```python
from build123d import *

# Parameters (mm, degrees)
BASPROSKE_W                  = 8
BASPROSKE_H                  = 13
TOOTHCUT_DEPTH               = 21.049937656
TEETHCUTS_COUNT              = 11
TEETHCUTS_ANGLE              = 327.272727273
BORSKE_R                     = 0.4
BORE_DEPTH                   = 50.0000508
ESTRUSIONE_ESTRUSIONE1_START = 10
SCHIZZO2_R                   = 13
ESTRUSIONE_ESTRUSIONE1_DEPTH = 10
TAGLIO_ESTRUSIONE1_DEPTH     = 14
FORO_PER_VITE_M3_1_D         = 4.2
FORO_PER_VITE_M3_1_DEPTH     = 9
FORO_PER_VITE_M3_1_TIP       = 1.2618073
SCHIZZO5_R                   = 11
TAGLIO_ESTRUSIONE2_DEPTH     = 2


with BuildPart() as part:
    # BasProSke → Base-Revolve (revolve)
    with BuildSketch(Plane(origin=(0, 0, 0), x_dir=(1, 0, 0), z_dir=(0, 1, 0)), mode=Mode.PRIVATE) as base_revolve_sk:
        with Locations((4, 6.5)):
            Rectangle(BASPROSKE_W, BASPROSKE_H)
    revolve(base_revolve_sk.sketch.rotate(Axis((-10, 0, 0), (1, 0, 0)), 180), axis=Axis((-10, 0, 0), (1, 0, 0)))

    # TooCutSke → ToothCut (cut, through all)
    with BuildSketch(Plane(origin=(0, 0, 0), x_dir=(0, 0, -1), z_dir=(1, 0, 0))):
        with BuildLine():
            ThreePointArc((1.139858048, 8.422216135), (0, 8.499), (-1.139858048, 8.422216135))
            ThreePointArc((-1.139858048, 8.422216135), (-1.658602184, 10.826907356), (-3.387115532, 12.577300725))
            ThreePointArc((-3.387115532, 12.577300725), (0, 13.0254), (3.387115532, 12.577300725))
            ThreePointArc((3.387115532, 12.577300725), (1.658602184, 10.826907356), (1.139858048, 8.422216135))
        make_face()
    toothcut = extrude(amount=TOOTHCUT_DEPTH, mode=Mode.SUBTRACT)

    # TeethCuts: ToothCut ×11 about axis
    teethcuts_axis = Axis((-10, 0, 0), (1, 0, 0))
    for i in range(1, TEETHCUTS_COUNT):
        add(toothcut.rotate(teethcuts_axis, i * TEETHCUTS_ANGLE / (TEETHCUTS_COUNT - 1)), mode=Mode.SUBTRACT)

    # BorSke → Bore (cut, symmetric)
    with BuildSketch(Plane(origin=(0, 0, 0), x_dir=(0, 0, -1), z_dir=(1, 0, 0))):
        with Locations(Location((0, 0, 0), (0, 0, 180))):
            Circle(BORSKE_R)
    extrude(amount=BORE_DEPTH, both=True, mode=Mode.SUBTRACT)

    # Schizzo2 → Estrusione-Estrusione1 (add)
    with BuildSketch(Plane(origin=(8, 0, 0), x_dir=(0, 0, -1), z_dir=(1, 0, 0)).offset(ESTRUSIONE_ESTRUSIONE1_START)):
        with Locations(Location((0, 0, 0), (0, 0, 173.223714884))):
            Circle(SCHIZZO2_R)
    extrude(amount=-ESTRUSIONE_ESTRUSIONE1_DEPTH)

    # Schizzo1 → Taglio-Estrusione1 (cut)
    with BuildSketch(Plane(origin=(18, 0, 0), x_dir=(0, 0, -1), z_dir=(1, 0, 0))):
        with BuildLine():
            Line((-1.5, 2), (1.5, 2))
            ThreePointArc((1.5, 2), (0, -2.5), (-1.5, 2))
        make_face()
    extrude(amount=-TAGLIO_ESTRUSIONE1_DEPTH, mode=Mode.SUBTRACT)

    # Foro per Vite M3-1
    with Locations(Plane(origin=(18, 0, 0), x_dir=(0, 0, -1), z_dir=(1, 0, 0))):
        with Locations((0, 8), (8, 0), (0, -8), (-8, 0)):
            Hole(FORO_PER_VITE_M3_1_D / 2, depth=FORO_PER_VITE_M3_1_DEPTH)
            with Locations((0, 0, -(FORO_PER_VITE_M3_1_DEPTH + FORO_PER_VITE_M3_1_TIP / 2))):  # 118° drill point
                Cone(0, FORO_PER_VITE_M3_1_D / 2, FORO_PER_VITE_M3_1_TIP, mode=Mode.SUBTRACT)

    # Schizzo5 → Taglio-Estrusione2 (cut)
    with BuildSketch(Plane(origin=(18, 0, 0), x_dir=(0, 0, -1), z_dir=(1, 0, 0))):
        Circle(SCHIZZO5_R)
    extrude(amount=-TAGLIO_ESTRUSIONE2_DEPTH, mode=Mode.SUBTRACT)


solid = part.part
```
Check sheet for the modelled part. Datum: model origin and axes. Units: mm. Round coordinates to 2 decimals unless told otherwise and drop trailing zeros. Order: outer loops, then holes, each group sorted by start corner. A loop starts at its lowest first (then second) coordinate and runs counter-clockwise, first axis right, second up.
1) Go/stop test with flat-tipped pins: pin 1 Ø1 at (x, z) = (11.5, 5.5) entering from -Y; pin 2 Ø1.6 at (y, z) = (-11, -3) entering from -X; pin 3 Ø10 at (x, y) = (12.5, -7) entering from +Z. Record where each tip stops, or that it passes through.
2) Mould release check, pull along Y, two halves, no side actions. Record for faces 1 (the conical face through (7.96, 8.31, -0.2)), 2 (the conical face through (7.96, -7.69, -0.2)): +Y half, -Y half, draft (parallel to the pull), parting line (faces both ways), or undercut.
3) Scan lines: line 1 (Y direction, x = 10.5, z = 0); line 2 (Z direction, x = 13.5, y = 0); line 3 (Y direction, x = 17.5, z = 0). Record each from-to range of solid material in increasing order.
4) Section check A-A (x = 13.5). Record the boundary of the cut face in (y, z), and give its area (3 significant figures).
Result:
1. pin 1: stops at y = -12
1. pin 2: stops at x = 8
1. pin 3: stops at z = 12.85
2. face 1: undercut
2. face 2: undercut
3. line 1: y = -13 to -10.1, -5.9 to -2.5, 2 to 5.9, 10.1 to 13
3. line 2: z = -13 to -10.1, -5.9 to -2.5, 2.5 to 5.9, 10.1 to 13
3. line 3: y = -13 to -11, 11 to 13
4. outline: circle Ø26 at (0, 0); hole circle Ø4.2 at (-8, 0); hole circle Ø4.2 at (0, -8); hole circle Ø4.2 at (0, 8); hole (2, -1.5) - (2, 1.5) arc R2.5 ccw (long way) to start; hole circle Ø4.2 at (8, 0)
4. area: 457 mm2
